Print and shaded views of the part. All mm, measured from the part's lowest x, y and z. A direction names the side the tool comes from. Round coordinates to 2 decimals unless told otherwise and drop trailing zeros. Loops run counter-clockwise (first coordinate to the right, second up) from the corner with the lowest first, then second, coordinate; pieces in that order, holes last. Notation, with made-up numbers: (89.25, 23.5) -> (137.25, 23.5) arc R24 ccw to (137.25, 45.5) -> close; hole circle Ø1 at (3.25, 86.25). An arc over 180 degrees is marked (long way). Use a Markdown table: item, result.
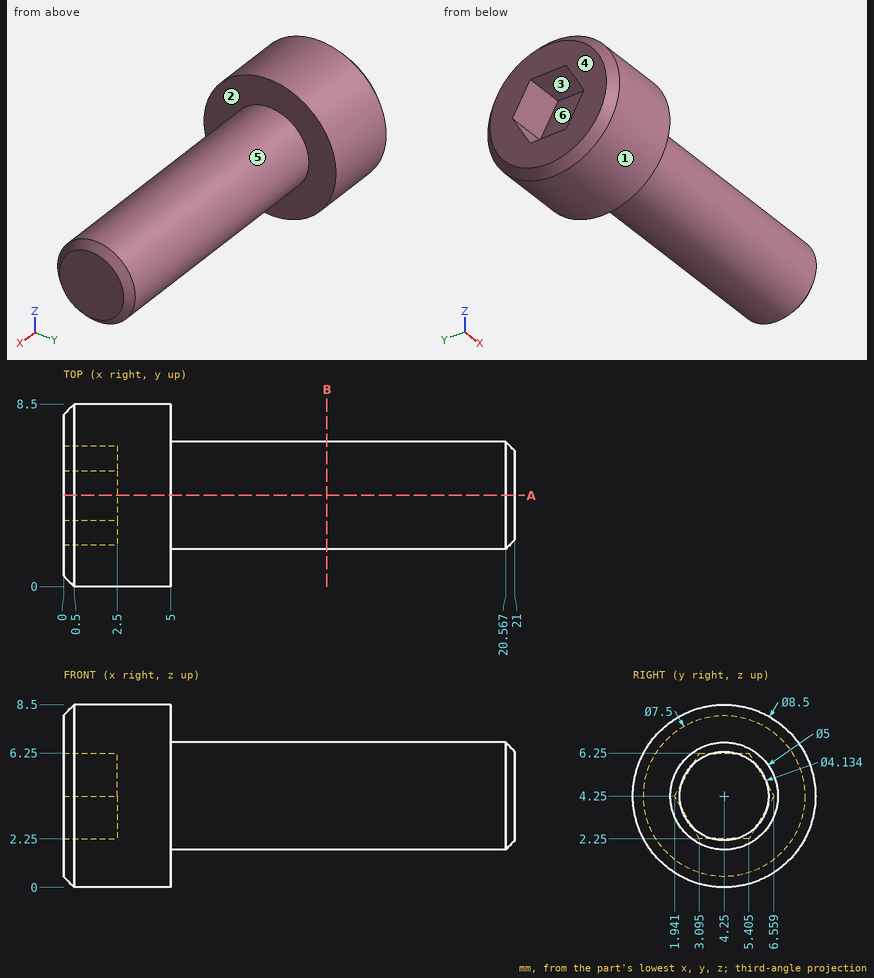
Q1. Drill centre lines: L1, parallel to X at y = 5.5, z = 5.75; L2, parallel to Z at x = 2, y = 0.5; L3, parallel to Y at x = 1.75, z = 5.75 (1 decimal). Where is each one in solid material? Low to high. Write a range as from..to.
Results list:
| item | result |
|---|---|
| L1 | x = 2.5..21 |
| L2 | z = 2.25..6.25 |
| L3 | y = 0.3..2.8, 5.7..8.2 |
Q2. Band-saw the part on A-A, the plane y = 4.25. Give the cut face in (x, z), plus the area to 3 significant figures.
Results list:
| item | result |
|---|---|
| outline | (0, 0.5) -> (0.5, 0) -> (5, 0) -> (5, 1.75) -> (20.57, 1.75) -> (21, 2.18) -> (21, 6.32) -> (20.57, 6.75) -> (5, 6.75) -> (5, 8.5) -> (0.5, 8.5) -> (0, 8) -> (0, 6.25) -> (2.5, 6.25) -> (2.5, 2.25) -> (0, 2.25) -> close |
| area | 112 mm² |
Q3. Flat gauge pins, fed straight in: pin 1 (1.5 mm diameter, centred on x = 14, y = 4, fed in from -Z); pin 2 (1.8 mm diameter, centred on x = 1.5, y = 4.5, fed in from +Z); pin 3 (2 mm diameter, centred on x = 14.5, z = 6, fed in from -Y) (1 decimal). Where does each tip first touch, or does it go through?
Results list:
| item | result |
|---|---|
| pin 1 | stops at z = 1.75 |
| pin 2 | stops at z = 8.5 |
| pin 3 | stops at y = 1.9 |
Q4. Pull direction Z, two halves, no side cores. Call the marked faces 4, 5 and 6: released by +Z, released by -Z, zero draft, split by the parting line, or undercut.
Results list:
| item | result |
|---|---|
| face 4 | zero draft |
| face 5 | split by the parting line |
| face 6 | undercut |
Q5. Tool access for the marked faces 1, 2 and 3: list every direction of +Z, -Z, +X, -X, +Y, -Y with a clear straight run to the whole face (end or side of a thin tool).
Results list:
| item | result |
|---|---|
| face 1 | +X, -X |
| face 2 | +X |
| face 3 | -X |
Q6. Band-saw the part on B-B, the plane x = 12.25. Give the cut face in (y, z), plus the area to 3 significant figures.
Results list:
| item | result |
|---|---|
| outline | circle Ø5 at (4.25, 4.25) |
| area | 19.6 mm² |
